```python
from build123d import *

# Parameters (mm, degrees)
SKETCH1_W           = 8
SKETCH1_H           = 27
SKETCH1_R           = 1.7
BOSS_EXTRUDE1_DEPTH = 5
CHAMFER1_SIZE       = 1.5
FILLET1_R           = 1
FILLET2_R           = 3


with BuildPart() as part:
    # Sketch1 → Boss-Extrude1 (new body)
    with BuildSketch(Plane.XY):
        Rectangle(SKETCH1_W, SKETCH1_H)
        with Locations((0, -9.5)):
            Circle(SKETCH1_R, mode=Mode.SUBTRACT)
    extrude(amount=BOSS_EXTRUDE1_DEPTH)

    # Chamfer1
    chamfer1_edges = [part.edges().sort_by_distance(p)[0] for p in [
        (0, -13.5, 0),
        (-4, 0, 0),
        (0, 13.5, 0),
        (4, 0, 0),
    ]]
    chamfer(chamfer1_edges, length=CHAMFER1_SIZE)

    # Fillet1
    fillet1_edges = [part.edges().sort_by_distance(p)[0] for p in [
        (-4, 0, 5),
        (0, -13.5, 5),
        (4, 0, 5),
        (0, 13.5, 5),
    ]]
    fillet(fillet1_edges, radius=FILLET1_R)

    # Fillet2
    # the kernel refuses this fillet: 3 mm, written as the material it takes off along each edge
    with BuildSketch(Plane(origin=(-1, 10.5, 5), x_dir=(0, 1, 0), z_dir=(1, 0, 0))) as fillet2_piece_1:
        with BuildLine():
            CenterArc((2, -1), 1, 0, 90)
            Line((3, -1), (3, 0))
            Line((3, 0), (2, 0))
        make_face()
    revolve(axis=Axis((-1, 10.5, 5), (0, 0, 1)), revolution_arc=90, mode=Mode.SUBTRACT)
    with BuildSketch(Plane(origin=(1, 10.5, 5), x_dir=(1, 0, 0), z_dir=(0, -1, 0))) as fillet2_piece_2:
        with BuildLine():
            CenterArc((2, -1), 1, 0, 90)
            Line((3, -1), (3, 0))
            Line((3, 0), (2, 0))
        make_face()
    revolve(axis=Axis((1, 10.5, 5), (0, 0, 1)), revolution_arc=90, mode=Mode.SUBTRACT)
    with BuildSketch(Plane(origin=(-1, -10.5, 5), x_dir=(-1, 0, 0), z_dir=(0, 1, 0))) as fillet2_piece_3:
        with BuildLine():
            CenterArc((2, -1), 1, 0, 90)
            Line((3, -1), (3, 0))
            Line((3, 0), (2, 0))
        make_face()
    revolve(axis=Axis((-1, -10.5, 5), (0, 0, 1)), revolution_arc=90, mode=Mode.SUBTRACT)
    with BuildSketch(Plane(origin=(1, -10.5, 5), x_dir=(0, -1, 0), z_dir=(-1, 0, 0))) as fillet2_piece_4:
        with BuildLine():
            CenterArc((2, -1), 1, 0, 90)
            Line((3, -1), (3, 0))
            Line((3, 0), (2, 0))
        make_face()
    revolve(axis=Axis((1, -10.5, 5), (0, 0, 1)), revolution_arc=90, mode=Mode.SUBTRACT)
    with BuildSketch(Plane(origin=(-6.5, 16, 4), x_dir=(0.816496580927726, 0.40824829046386274, 0.40824829046386324), z_dir=(0.5773502691896258, -0.5773502691896258, -0.5773502691896258)), Plane(origin=(-6.5, -16, 4), x_dir=(-0.4082482904638628, 0.816496580927726, 0.40824829046386335), z_dir=(0.5773502691896257, 0.5773502691896258, -0.5773502691896257))) as fillet2_piece_5:
        with BuildLine():
            CenterArc((FILLET2_R * 0.57735026919, FILLET2_R), FILLET2_R, 210, 60)
            Line((-FILLET2_R * 0.288675134595, FILLET2_R * 0.5), (0, 0))
            Line((0, 0), (FILLET2_R * 0.57735026919, 0))
        make_face()
    extrude(amount=11.258330249, mode=Mode.SUBTRACT)
    with BuildSketch(Plane(origin=(6.5, 16, 4), x_dir=(-0.8164965809277261, 0.4082482904638628, 0.4082482904638633), z_dir=(-0.5773502691896258, -0.5773502691896258, -0.5773502691896258)), Plane(origin=(6.5, -16, 4), x_dir=(0.4082482904638627, 0.8164965809277261, 0.4082482904638632), z_dir=(-0.5773502691896258, 0.5773502691896257, -0.5773502691896258))) as fillet2_piece_6:
        with BuildLine():
            CenterArc((FILLET2_R * 0.57735026919, -FILLET2_R), FILLET2_R, 90, 60)
            Line((-FILLET2_R * 0.288675134595, -FILLET2_R * 0.5), (0, 0))
            Line((0, 0), (FILLET2_R * 0.57735026919, 0))
        make_face()
    extrude(amount=11.258330249, mode=Mode.SUBTRACT)
    with BuildSketch(Plane(origin=(-4, -13.5, -6), x_dir=(0, 1, 0), z_dir=(0, 0, 1)), Plane(origin=(-4, 13.5, -6), x_dir=(1, 0, 0), z_dir=(0, 0, 1))) as fillet2_piece_7:
        with BuildLine():
            CenterArc((FILLET2_R, -FILLET2_R), FILLET2_R, 90, 90)
            Line((0, -FILLET2_R), (0, 0))
            Line((0, 0), (FILLET2_R, 0))
        make_face()
    extrude(amount=11, mode=Mode.SUBTRACT)
    with BuildSketch(Plane(origin=(4, -13.5, -6), x_dir=(0, 1, 0), z_dir=(0, 0, 1)), Plane(origin=(4, 13.5, -6), x_dir=(-1, 0, 0), z_dir=(0, 0, 1))) as fillet2_piece_8:
        with BuildLine():
            CenterArc((FILLET2_R, FILLET2_R), FILLET2_R, 180, 90)
            Line((0, FILLET2_R), (0, 0))
            Line((0, 0), (FILLET2_R, 0))
        make_face()
    extrude(amount=11, mode=Mode.SUBTRACT)


solid = part.part
```
The listing builds one solid part. Answer for the finished solid, in the listing's coordinates (mm). Coordinates: 2 decimals unless noted, no trailing zeros. Write each loop counter-clockwise with the first axis right and the second up, starting at its lowest first coordinate (ties: lowest second). Pieces come first, ordered by that corner, then holes. Notation, with made-up numbers: (15.25, 42.25) - (73.25, 42.25) arc R22 cw to (73.25, 74.25) - close; hole circle Ø10 at (52, 70.25). An arc over 180 degrees is marked (long way). One line per item, written item: value.
1) Find section A-A (y = -9.5). Give the vertices of the cut face in (x, z), and give its area (3 significant figures).
Geometry check:
outline: (-4, 1.5) - (-2.5, 0) - (-1.7, 0) - (-1.7, 5) - (-3, 5) arc R1 ccw to (-4, 4) - close; (1.7, 0) - (2.5, 0) - (4, 1.5) - (4, 4) arc R1 ccw to (3, 5) - (1.7, 5) - close
area: 20.3 mm2
2) Consider line 1 along Y through (x, z) = (0, 2.7); line 2 along X through (y, z) = (-4.75, 0.5); line 3 along Y through (x, z) = (0.5, 3.5). Determine where each line is inside the solid, lowest interval first. Write a range as from..to.
Geometry check:
line 1: y = -13.5..-11.2, -7.8..13.5
line 2: x = -3..3
line 3: y = -13.5..-11.12, -7.88..13.5
3) Find section B-B (x = 0). Give the vertices of the cut face in (y, z).
Geometry check:
outline: (-13.5, 1.5) - (-12, 0) - (-11.2, 0) - (-11.2, 5) - (-12.5, 5) arc R1 ccw to (-13.5, 4) - close; (-7.8, 0) - (12, 0) - (13.5, 1.5) - (13.5, 4) arc R1 ccw to (12.5, 5) - (-7.8, 5) - close
4) This flat-tipped pin is pushed along its axis until it touches: pin 1 Ø2 at (x, z) = (3, 3.5) entering from -Y. Where does it stop, or does it pass through?
Geometry check:
pin 1: stops at y = -13.33
5) Find section C-C (z = 4.5). Give the vertices of the cut face in (x, y).
Geometry check:
outline: (-3.87, -10.5) arc R2.87 ccw to (-1, -13.37) - (1, -13.37) arc R2.87 ccw to (3.87, -10.5) - (3.87, 10.5) arc R2.87 ccw to (1, 13.37) - (-1, 13.37) arc R2.87 ccw to (-3.87, 10.5) - close; hole circle Ø3.4 at (0, -9.5)
6) Find section D-D (y = -4.25). Give the vertices of the cut face in (x, z).
Geometry check:
outline: (-4, 1.5) - (-2.5, 0) - (2.5, 0) - (4, 1.5) - (4, 4) arc R1 ccw to (3, 5) - (-3, 5) arc R1 ccw to (-4, 4) - close
